```python
from build123d import *

# Parameters (mm, degrees)
F0_R     = 16.05
F1_DEPTH = 12
F3_DEPTH = 25
F5_DEPTH = 25


# Not quite as in the source:
# - a feature names something its author has since deleted; it is built from what else it names


with BuildPart() as f1:
    # F0 (on Top) → F1 (new body)
    with BuildSketch(Plane.XY):
        with BuildLine():
            ThreePointArc((0, -18.05), (12.7632774004, -12.7632774004), (18.05, 0))
            ThreePointArc((18.05, 0), (12.7632774004, 12.7632774004), (0, 18.05))
            ThreePointArc((0, 18.05), (-18.05, 0), (0, -18.05))
        make_face()
        Circle(F0_R, mode=Mode.SUBTRACT)
        with BuildLine():
            ThreePointArc((0, 18.05), (12.7632774004, 12.7632774004), (18.05, 0))
            ThreePointArc((18.05, 0), (12.7632774004, -12.7632774004), (0, -18.05))
            Line((0, -18.05), (16.7152378708, -18.05))
            Line((16.7152378708, -18.05), (16.7, -25))
            Line((16.7, -25), (19.7, -25))
            Line((19.7, -25), (19.7, 0))
            Line((19.7, 0), (19.7, 25))
            Line((19.7, 25), (16.7, 25))
            Line((16.7, 25), (16.7152378708, 18.05))
            Line((16.7152378708, 18.05), (0, 18.05))
        make_face()
    extrude(amount=F1_DEPTH)

    # F2 (on face) → F3 (cut)
    with BuildSketch(Plane(origin=(16.754731944, -0.0367347397, 0), x_dir=(-0.0021924941, -0.9999975965, 0), z_dir=(-0.9999975965, 0.0021924941, 0))):
        with BuildLine():
            ThreePointArc((23.7358004302, 5.5), (20.3215868678, 6.9142135624), (21.7358004302, 3.5))
            Line((21.7358004302, 3.5), (21.7358004302, 5.5))
            Line((21.7358004302, 5.5), (23.7358004302, 5.5))
        make_face()
        with BuildLine():
            Line((21.7358004302, 5.5), (21.7358004302, 3.5))
            ThreePointArc((21.7358004302, 3.5), (23.1500139926, 4.0857864376), (23.7358004302, 5.5))
            Line((23.7358004302, 5.5), (21.7358004302, 5.5))
        make_face()
    extrude(amount=-F3_DEPTH, mode=Mode.SUBTRACT)

    # F4 (on face) → F5 (cut)
    with BuildSketch(Plane(origin=(16.754731944, 0.0367347397, 0), x_dir=(0.0021924941, -0.9999975965, 0), z_dir=(-0.9999975965, -0.0021924941, 0))):
        with BuildLine():
            Line((-21.5104483068, 6.5), (-21.5104483068, 8.5))
            ThreePointArc((-21.5104483068, 8.5), (-22.9246618692, 7.9142135624), (-23.5104483068, 6.5))
            Line((-23.5104483068, 6.5), (-21.5104483068, 6.5))
        make_face()
        with BuildLine():
            ThreePointArc((-19.5104483068, 6.5), (-20.0962347444, 7.9142135624), (-21.5104483068, 8.5))
            Line((-21.5104483068, 8.5), (-21.5104483068, 6.5))
            Line((-21.5104483068, 6.5), (-23.5104483068, 6.5))
            ThreePointArc((-23.5104483068, 6.5), (-21.5104483068, 4.5), (-19.5104483068, 6.5))
        make_face()
    extrude(amount=-F5_DEPTH, mode=Mode.SUBTRACT)


solid = f1.part
```
Can you work these out from the model? Positions are in its coordinate system, mm. A direction names the side the tool comes from. Coordinates: 2 decimals unless noted, no trailing zeros. Loops run counter-clockwise (first coordinate to the right, second up) from the corner with the lowest first, then second, coordinate; pieces in that order, holes last. Notation, with made-up numbers: (3.25, 26) -> (30.25, 26) arc R18 ccw to (30.25, 34) -> close; hole circle Ø8 at (72.25, 61). An arc over 180 degrees is marked (long way). Put each result on its own line as item: value. Start each with the question number.
Q1. For faces 1 (the face through (19.7, 0, 6)), 2 (the face through (8, -18.05, 6)), 3 (the face through (8, 18.05, 6)), which set-ups out of +Z, -Z, +X, -X, +Y, -Y let a thin tool reach every point of the face, with its end or its side?
Q2. Thinking about a two-plate mould opening in Y: for faces 4 (the face through (16.12, -1.74, 12)), 5 (the face through (-12.737, -9.766, 5.916)), 6 (the face through (18, -25, 6)), which applies, pulls with the +Y half, pulls with the -Y half, needs draft (parallel to the pull), parting line crosses it, or undercut?
Q3. I want a section at A-A (y = 0). Write out the boundary of the cut face in (x, z).
Q4. If I drill on line 1 (Y direction, x = 5.5, z = 2); line 2 (Y direction, x = -13.5, z = 7.75); line 3 (X direction, y = 6, z = 3), over which ranges is the centre line in solid material (lowest first)? Write a range as [from, to].
Q5. I want a section at B-B (x = -4.5). Write out the boundary of the cut face in (y, z).
Q6. I'm going to push flat-ended pins straight in: P1, Ø6, axis at y = -16.5, z = 8.5, coming from the -X side; P2, Ø1.5, axis at y = 3, z = 10.5, coming from the -X side; P3, Ø8, axis at x = -7.5, y = -6.5, coming from the +Z side; P4, Ø1, axis at x = 15, z = 1.5, coming from the -Y side. Where does each tip first touch, or does it pass through?
Taken from the geometry:
1. face 1: +Z, -Z, +X, +Y, -Y
1. face 2: +Z, -Z, -X, -Y
1. face 3: +Z, -Z, -X, +Y
2. face 4: needs draft
2. face 5: undercut
2. face 6: pulls with the -Y half
3. outline: (-18.05, 0) -> (-16.05, 0) -> (-16.05, 12) -> (-18.05, 12) -> close; (16.05, 0) -> (19.7, 0) -> (19.7, 12) -> (16.05, 12) -> close
4. line 1: y = [-18.05, -15.08], [15.08, 18.05]
4. line 2: y = [-11.98, -8.68], [8.68, 11.98]
4. line 3: x = [-17.02, -14.89], [14.89, 19.7]
5. outline: (-17.48, 0) -> (-15.41, 0) -> (-15.41, 12) -> (-17.48, 12) -> close; (15.41, 0) -> (17.48, 0) -> (17.48, 12) -> (15.41, 12) -> close
6. P1: stops at x = -11.98
6. P2: stops at x = -17.91
6. P3: passes through
6. P4: stops at y = -18.05
